```python
from build123d import *

# Parameters (mm, degrees)
EXTRUDE_THIN1_DEPTH = 0.2
FILLET2_R           = 0.05


with BuildPart() as part:
    # Sketch1 → Extrude-Thin1 (new, symmetric)
    with BuildSketch(Plane(origin=(0, 0, 0), x_dir=(0, 0, -1), z_dir=(1, 0, 0))):
        with BuildLine():
            Line((1.5, 0), (0.4, 0))
            ThreePointArc((0.4, 0), (0.117157288, 0.117157288), (0, 0.4))
            Line((0, 0.4), (0, 1.5))
            ThreePointArc((0, 1.5), (-0.029289322, 1.570710678), (-0.1, 1.6))
            Line((-0.1, 1.6), (-2.4, 1.6))
            Line((-2.4, 1.6), (-4.511931163, 1.853790806))
            ThreePointArc((-4.511931163, 1.853790806), (-4.570232229, 1.88189058), (-4.599115742, 1.939807369))
            ThreePointArc((-4.599115742, 1.939807369), (-4.774219375, 2.173964421), (-5.065441937, 2.147883256))
            Line((-5.065441937, 2.147883256), (-5.843673678, 1.617372248))
            ThreePointArc((-5.843673678, 1.617372248), (-5.870527769, 1.604441706), (-5.9, 1.6))
            Line((-5.9, 1.6), (-6.9, 1.6))
            Line((-6.9, 1.6), (-6.9, 1.9))
            Line((-6.9, 1.9), (-5.961684297, 1.9))
            Line((-5.961684297, 1.9), (-5.234420904, 2.395766512))
            ThreePointArc((-5.234420904, 2.395766512), (-4.728210685, 2.475926357), (-4.344765926, 2.135860917))
            Line((-4.344765926, 2.135860917), (-2.382039107, 1.9))
            Line((-2.382039107, 1.9), (-0.1, 1.9))
            ThreePointArc((-0.1, 1.9), (0.182842712, 1.782842712), (0.3, 1.5))
            Line((0.3, 1.5), (0.3, 0.4))
            ThreePointArc((0.3, 0.4), (0.329289322, 0.329289322), (0.4, 0.3))
            Line((0.4, 0.3), (1.5, 0.3))
            Line((1.5, 0.3), (1.5, 0))
        make_face()
    extrude(amount=EXTRUDE_THIN1_DEPTH, both=True)

    # Sketch3 → Loft1 section 0
    with BuildSketch(Plane(origin=(0, 0.35, 0), x_dir=(1, 0, 0), z_dir=(0, 1, 0))):
        with BuildLine():
            Line((0.2, 1.6), (0.2, 0.6))
            ThreePointArc((0.2, 0.6), (0, 0.4), (-0.2, 0.6))
            Line((-0.2, 0.6), (-0.2, 1.6))
            ThreePointArc((-0.2, 1.6), (0, 1.8), (0.2, 1.6))
        make_face()
    # Sketch2 → Loft1 section 1
    with BuildSketch(Plane(origin=(0, -0.05, 0), x_dir=(1, 0, 0), z_dir=(0, 1, 0))):
        with BuildLine():
            Line((0.25, 2.25), (0.25, 0.25))
            ThreePointArc((0.25, 0.25), (0, 0), (-0.25, 0.25))
            Line((-0.25, 0.25), (-0.25, 2.25))
            ThreePointArc((-0.25, 2.25), (0, 2.5), (0.25, 2.25))
        make_face()
    loft()

    # Fillet2
    fillet2_edges = [part.edges().sort_by_distance(p)[0] for p in [
        (0, 0.35, -1.8),
        (-0.2, 0.35, -1.1),
        (0, 0.35, -0.4),
        (0.2, 0.35, -1.1),
    ]]
    fillet(fillet2_edges, radius=FILLET2_R)


solid = part.part
```
Could you check a few things on this model? Use its own coordinates, in mm. Coordinates: 2 decimals unless noted, no trailing zeros. Write each loop counter-clockwise with the first axis right and the second up, starting at its lowest first coordinate (ties: lowest second). Pieces come first, ordered by that corner, then holes. Notation, with made-up numbers: (-4.75, 30) -> (33.25, 30) arc R29 cw to (33.25, 64) -> close; hole circle Ø7 at (50, -14.5). An arc over 180 degrees is marked (long way). Write item = value, one per line. Start each with the question number.
(1) I want a section at A-A (y = 1.4). Please give me the cut outline in (x, z), plus the area to 3 significant figures.
(2) I want a section at B-B (z = 2). Please give me the cut outline in (x, y).
(3) I need wall thicknesses on line 1 (Z direction, x = 0.05, y = 1.35); line 2 (Y direction, x = 0, z = 0.25); line 3 (Y direction, x = -0.1, z = -1.25). Which ranges of each line are inside material? Lowest first, please. Write a range as [from, to].
Result set:
q1.outline = (-0.2, -0.3) -> (0.2, -0.3) -> (0.2, 0) -> (-0.2, 0) -> close
q1.area = 0.120 mm2
q2.outline = (-0.2, 1.6) -> (0.2, 1.6) -> (0.2, 1.9) -> (-0.2, 1.9) -> close
q3.line_1 = [-0.3, 0]
q3.line_2 = [1.6, 1.9]
q3.line_3 = [-0.05, 0.35]
